Check sheet for the drawn part. Datum: minimum x, y, z corner. Units: mm. Give positions to 0.01 mm unless a question says otherwise; leave off trailing zeros. Loops run counter-clockwise (first coordinate to the right, second up) from the corner with the lowest first, then second, coordinate; pieces in that order, holes last.
1. Cross-section at A-A, the plane z = 133.35. Record the cut outline in (x, y) (1 decimal), plus the area to 3 significant figures.
2. Release check for a two-part mould opening along X. For the marked faces 1 and 2 record: +X half, -X half, draft (parallel to the pull), parting line (faces both ways), or undercut.
3. Material ranges on L1, parallel to X at y = 16, z = 206 (1 decimal); L2, parallel to X at y = 1.45, z = 228.6 (1 decimal); L3, parallel to Z at x = 9, y = 3, recorded low to high.
4. Cross-section at B-B, the plane y = 10.25. Record the cut outline in (x, z) (1 decimal), plus the area to 3 significant figures.
5. Cross-section at D-D, the plane z = 299. Record the cut outline in (x, y) (1 decimal), plus the area to 3 significant figures.
6. Cross-section at C-C, the plane x = 37. Record the cut outline in (y, z) (1 decimal).
7. Go/stop test with flat-tipped pins: pin 1 Ø10 at (x, z) = (40.5, 51.5) entering from +Y (1 decimal); pin 2 Ø17 at (x, z) = (18.73, 260.35) entering from +Y. Record where each tip stops, or that it passes through.
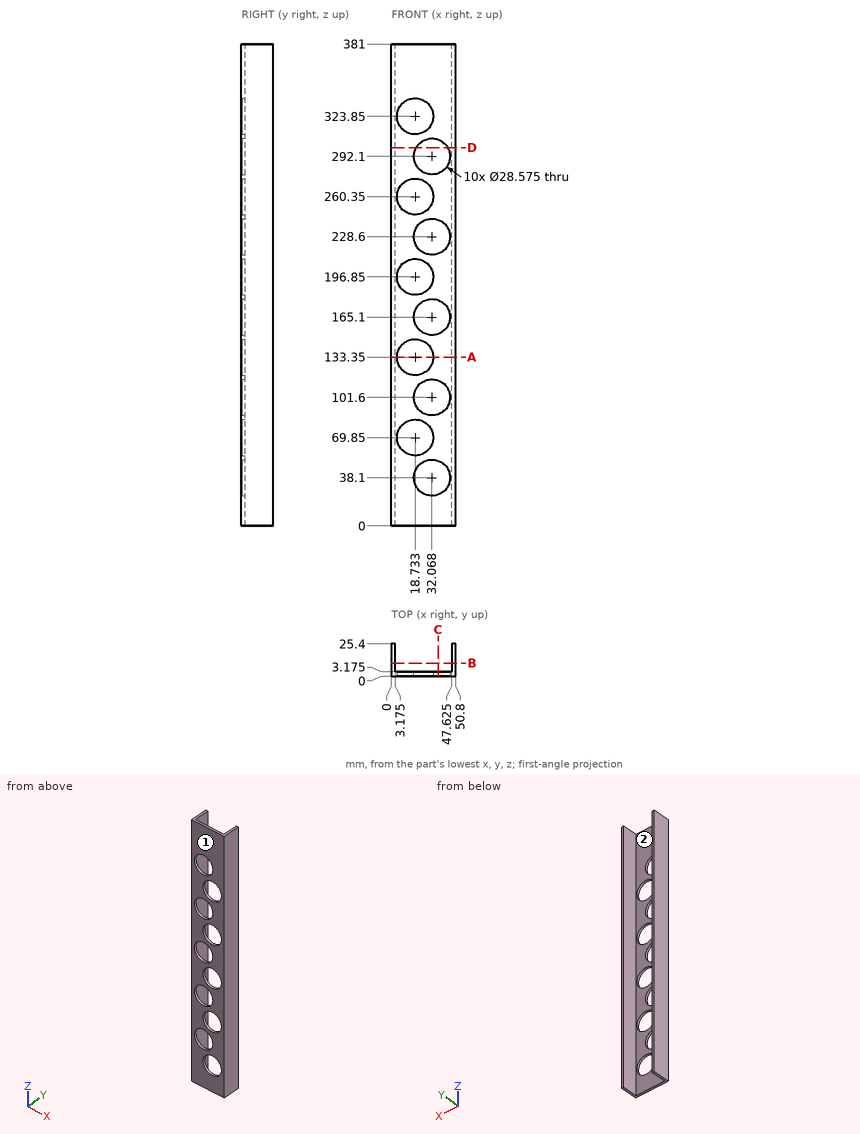
Result:
1. outline: (0, 0) - (4.4, 0) - (4.4, 3.2) - (3.2, 3.2) - (3.2, 25.4) - (0, 25.4) - close; (33, 0) - (50.8, 0) - (50.8, 25.4) - (47.6, 25.4) - (47.6, 3.2) - (33, 3.2) - close
1. area: 212 mm2
2. face 1: draft
2. face 2: undercut
3. L1: x = 0 to 3.2, 47.6 to 50.8
3. L2: x = 0 to 17.8, 46.4 to 50.8
3. L3: z = 0 to 59.39, 80.31 to 122.89, 143.81 to 186.39, 207.31 to 249.89, 270.81 to 313.39, 334.31 to 381
4. outline: (0, 0) - (3.2, 0) - (3.2, 381) - (0, 381) - close; (47.6, 0) - (50.8, 0) - (50.8, 381) - (47.6, 381) - close
4. area: 2,420 mm2
5. outline: (0, 0) - (19.6, 0) - (19.6, 3.2) - (3.2, 3.2) - (3.2, 25.4) - (0, 25.4) - close; (44.6, 0) - (50.8, 0) - (50.8, 25.4) - (47.6, 25.4) - (47.6, 3.2) - (44.6, 3.2) - close
5. area: 223 mm2
6. outline: (0, 0) - (3.2, 0) - (3.2, 24.7) - (0, 24.7) - close; (0, 51.5) - (3.2, 51.5) - (3.2, 88.2) - (0, 88.2) - close; (0, 115) - (3.2, 115) - (3.2, 151.7) - (0, 151.7) - close; (0, 178.5) - (3.2, 178.5) - (3.2, 215.2) - (0, 215.2) - close; (0, 242) - (3.2, 242) - (3.2, 278.7) - (0, 278.7) - close; (0, 305.5) - (3.2, 305.5) - (3.2, 381) - (0, 381) - close
7. pin 1: stops at y = 3.2
7. pin 2: passes through
